The model under review builds one solid part; all positions refer to its coordinate system, in mm. A direction names the side the tool comes from. Give positions to 0.01 mm unless a question says otherwise; leave off trailing zeros. Order: outer loops, then holes, each group sorted by start corner. A loop starts at its lowest first (then second) coordinate and runs counter-clockwise, first axis right, second up. Notation, with made-up numbers: (61, 36.5) - (106, 36.5) arc R9 ccw to (106, 50.5) - close; hole circle Ø1 at (-26, -21.5). An arc over 180 degrees is marked (long way). Use CSV: the item, a comma, the result in double quotes.
```python
from build123d import *

# Parameters (mm, degrees)
EXTRUDE_1_DEPTH          = 7
SKETCH_2_R               = 3
CUT_EXTRUDE_1_DEPTH      = 8
MIRROR_2_COPY_1_SKETCH_R = 3
MIRROR_2_COPY_1_DEPTH    = 8
SKETCH_3_R               = 13
EXTRUDE_2_DEPTH          = 35
EXTRUDE_3_DEPTH          = 6
SKETCH_5_R               = 9
CUT_EXTRUDE_2_DEPTH      = 10
SKETCH_6_R               = 6
CUT_EXTRUDE_3_DEPTH      = 39
EXTRUDE_4_REACH          = 36
CUT_EXTRUDE_4_REACH      = 36
SKETCH_8_R               = 6
EXTRUDE_6_DEPTH          = 6


with BuildPart() as part:
    # 草图1 → 凸台-拉伸1 (new body)
    with BuildSketch(Plane(origin=(0, 0, 0), x_dir=(1, 0, 0), z_dir=(0, 1, 0))):
        with BuildLine():
            Line((-27.110883423, 17), (27.110883423, 17))
            ThreePointArc((27.110883423, 17), (32, 0), (27.110883423, -17))
            Line((27.110883423, -17), (-27.110883423, -17))
            ThreePointArc((-27.110883423, -17), (-32, 0), (-27.110883423, 17))
        make_face()
    extrude(amount=EXTRUDE_1_DEPTH)

    # 草图2 → 切除-拉伸1 (cut, through all)
    with BuildSketch(Plane(origin=(0, 7, 0), x_dir=(1, 0, 0), z_dir=(0, 1, 0))):
        with Locations((-20, -12)):
            Circle(SKETCH_2_R)
    cut_extrude_1 = extrude(amount=-CUT_EXTRUDE_1_DEPTH, mode=Mode.SUBTRACT)

    # 镜向1: 切除-拉伸1 across plane
    add(cut_extrude_1.mirror(Plane(origin=(0, 0, 0), x_dir=(0, 0, 1), z_dir=(1, 0, 0))), mode=Mode.SUBTRACT)

    # 镜向2: 切除-拉伸1 across plane
    add(cut_extrude_1.mirror(Plane.XY), mode=Mode.SUBTRACT)

    # 镜向2 copy 1 sketch → 镜向2 copy 1 (cut, through all)
    with BuildSketch(Plane(origin=(0, 7, 0), x_dir=(-1, 0, 0), z_dir=(0, 1, 0))):
        with Locations((-20, -12)):
            Circle(MIRROR_2_COPY_1_SKETCH_R)
    extrude(amount=-MIRROR_2_COPY_1_DEPTH, mode=Mode.SUBTRACT)

    # 草图3 → 凸台-拉伸2 (add)
    with BuildSketch(Plane(origin=(0, 7, 0), x_dir=(1, 0, 0), z_dir=(0, 1, 0))):
        Circle(SKETCH_3_R)
    extrude(amount=EXTRUDE_2_DEPTH)

    # 草图4 → 凸台-拉伸3 (add)
    with BuildSketch(Plane(origin=(0, 42, 0), x_dir=(1, 0, 0), z_dir=(0, 1, 0))):
        with BuildLine():
            Line((-14.736938996, 13.5), (14.736938996, 13.5))
            ThreePointArc((14.736938996, 13.5), (19.985679147, 0), (14.736938996, -13.5))
            Line((14.736938996, -13.5), (-14.736938996, -13.5))
            ThreePointArc((-14.736938996, -13.5), (-19.985679147, 0), (-14.736938996, 13.5))
        make_face()
    extrude(amount=EXTRUDE_3_DEPTH)

    # 草图5 → 切除-拉伸2 (cut)
    with BuildSketch(Plane(origin=(0, 48, 0), x_dir=(1, 0, 0), z_dir=(0, 1, 0))):
        Circle(SKETCH_5_R)
    extrude(amount=-CUT_EXTRUDE_2_DEPTH, mode=Mode.SUBTRACT)

    # 草图6 → 切除-拉伸3 (cut, through all)
    with BuildSketch(Plane(origin=(0, 38, 0), x_dir=(1, 0, 0), z_dir=(0, 1, 0))):
        Circle(SKETCH_6_R)
    extrude(amount=-CUT_EXTRUDE_3_DEPTH, mode=Mode.SUBTRACT)

    # 草图7 → 凸台-拉伸4 (add, up to next)
    with BuildSketch(Plane.XY.offset(17), mode=Mode.PRIVATE) as extrude_4_sk1:
        with BuildLine():
            Line((-9, 7), (-9, 23))
            ThreePointArc((-9, 23), (0, 32), (9, 23))
            Line((9, 23), (9, 7))
            Line((9, 7), (-9, 7))
        make_face()
    extrude_4_tool1 = extrude(extrude_4_sk1.sketch, amount=-EXTRUDE_4_REACH, mode=Mode.PRIVATE) - part.part
    add(extrude_4_tool1.solids().sort_by_distance((0, 18.621751, 17))[0])

    # 草图8 → 切除-拉伸4 (cut, up to next)
    with BuildSketch(Plane.XY.offset(17), mode=Mode.PRIVATE) as cut_extrude_4_sk1:
        with Locations((0, 20.461682424)):
            Circle(SKETCH_8_R)
    cut_extrude_4_tool1 = extrude(cut_extrude_4_sk1.sketch, amount=-CUT_EXTRUDE_4_REACH, mode=Mode.PRIVATE) & part.part
    add(cut_extrude_4_tool1.solids().sort_by_distance((0, 20.461682, 17))[0], mode=Mode.SUBTRACT)

    # 草图10 → 凸台-拉伸6 (add, symmetric)
    with BuildSketch(Plane.XY):
        Polygon((-10.493273041, 6.945714178), (-22.343826616, 7), (-14.941545846, 22.874242338), (-10.666084354, 32.042999097), align=None)
    extrude_6 = extrude(amount=EXTRUDE_6_DEPTH, both=True)

    # 镜向4: 凸台-拉伸6 across plane
    add(extrude_6.mirror(Plane(origin=(0, 0, 0), x_dir=(0, 0, 1), z_dir=(1, 0, 0))))


solid = part.part
```
Item 1: Take a section at A-A, the plane x = 0. Give the boundary of the cut face in (y, z).
Results list:
outline,"(0, -17) - (7, -17) - (7, -13) - (42, -13) - (42, -13.5) - (48, -13.5) - (48, -9) - (38, -9) - (38, -6) - (0, -6) - close; (0, 6) - (14.46, 6) - (14.46, 17) - (0, 17) - close; (26.46, 6) - (38, 6) - (38, 9) - (48, 9) - (48, 13.5) - (42, 13.5) - (42, 13) - (32, 13) - (32, 17) - (26.46, 17) - close"
Item 2: Clearance check with flat-ended pins moving along their axes: pin 1 (2 mm diameter, centred on x = 12.5, y = 28.5, fed in from +Z); pin 2 (1.5 mm diameter, centred on y = 36.5, z = -3, fed in from +X); pin 3 (3 mm diameter, centred on x = 3.5, y = 45, fed in from -Z). State where each tip first meets the part, or that it passes through.
Results list:
pin 1,"stops at z = 6.06"
pin 2,"stops at x = 12.8"
pin 3,"stops at z = -13.5"
Item 3: Tool access review of faces 5 (the face through (0, 45, 13.5)), 6 (the face through (0, 45, -13.5)), 7 (the face through (-19.985, 44.958, 0.208)), 8 (the face through (-9.58, 28.14, -8.79)), 9 (the face through (-14, 14, -6)): name each direction out of +Z, -Z, +X, -X, +Y, -Y from which nothing blocks a thin tool from reaching the whole face with its end or side.
Results list:
face 5,"+Z, +X, -X, +Y"
face 6,"-Z, +X, -X, +Y"
face 7,"-X, +Y"
face 8,"none"
face 9,"-Z, -X"
Item 4: Take a section at D-D, the plane y = 44. Give the boundary of the cut face in (x, z), and give its area (3 significant figures).
Results list:
outline,"(-14.74, -13.5) - (14.74, -13.5) arc R19.99 ccw to (14.74, 13.5) - (-14.74, 13.5) arc R19.99 ccw to start; hole circle Ø18 at (0, 0)"
area,"736 mm2"
Item 5: Wall thickness on L1, parallel to Z at x = 20, y = 2; L2, parallel to Y at x = 0, z = 11; L3, parallel to Z at x = 18, y = 3.5: over which ranges is each line inside the solid? List them lowest first.
Results list:
L1,"z = -17 to -15, -9 to 9, 15 to 17"
L2,"y = 0 to 14.46, 26.46 to 48"
L3,"z = -17 to -14.24, -9.76 to 9.76, 14.24 to 17"
Item 6: Mouldability with a two-part tool opening along Z and no side actions: class faces 1 (the face through (2, 38, 6)), 2 (the face through (9, 15, 13)), 3 (the face through (0, 3, -17)), 4 (the face through (23, 4, 12)) as pulls with the +Z half, pulls with the -Z half, needs draft (parallel to the pull), parting line crosses it, or undercut.
Results list:
face 1,"undercut"
face 2,"needs draft"
face 3,"pulls with the -Z half"
face 4,"undercut"
Item 7: Take a section at C-C, the plane z = 12. Give the boundary of the cut face in (x, y), and give its area (3 significant figures).
Results list:
outline,"(-29.66, 0) - (-23, 0) - (-23, 7) - (-29.66, 7) - close; (-17, 0) - (17, 0) - (17, 7) - (9, 7) - (9, 23) arc R9 ccw to (5, 30.48) - (5, 42) - (15.98, 42) - (15.98, 48) - (-15.98, 48) - (-15.98, 42) - (-5, 42) - (-5, 30.48) arc R9 ccw to (-9, 23) - (-9, 7) - (-17, 7) - close; (23, 0) - (29.66, 0) - (29.66, 7) - (23, 7) - close; hole circle Ø12 at (0, 20.46)"
area,"930 mm2"
Item 8: Take a section at B-B, the plane y = 5.5. Give the boundary of the cut face in (x, z), and give its area (3 significant figures).
Results list:
outline,"(-27.11, -17) - (27.11, -17) arc R32 ccw to (27.11, 17) - (-27.11, 17) arc R32 ccw to start; hole circle Ø6 at (-20, -12); hole circle Ø6 at (-20, 12); hole circle Ø12 at (0, 0); hole circle Ø6 at (20, -12); hole circle Ø6 at (20, 12)"
area,"1,840 mm2"
